from build123d import *

# Parameters (mm, degrees)
SKETCH2_OUTSIDE_W  = 34.928
SKETCH2_OUTSIDE_H  = 34.928
SKETCH2_OUTSIDE_R  = 3.81
CUT_EXTRUDE1_DEPTH = 0.5
CHAMFER1_SIZE2     = 2
CHAMFER1_SIZE      = 0.515


with BuildPart() as part:
    # Sketch1 → Revolve1 (revolve)
    with BuildSketch(Plane.XY, mode=Mode.PRIVATE) as revolve1_sk:
        with BuildLine():
            Line((0, 0), (64.25, 0))
            Line((64.25, 0), (64.25, 4.325))
            Line((64.25, 4.325), (56.25, 4.325))
            ThreePointArc((56.25, 4.325), (52.653126358, 4.994271197), (49.5377095, 6.9125))
            ThreePointArc((49.5377095, 6.9125), (46.422292643, 8.830728803), (42.825419001, 9.5))
            Line((42.825419001, 9.5), (9.5, 9.5))
            ThreePointArc((9.5, 9.5), (2.782485579, 6.717514421), (0, 0))
        make_face()
    revolve(revolve1_sk.sketch.rotate(Axis((71.903875566, 0, 0), (1, 0, 0)), 90), axis=Axis((71.903875566, 0, 0), (1, 0, 0)))

    # Sketch2 outside → Cut-Extrude1 (cut)
    with BuildSketch(Plane(origin=(64.25, 0, 0), x_dir=(0, 0, -1), z_dir=(1, 0, 0))):
        Rectangle(SKETCH2_OUTSIDE_W, SKETCH2_OUTSIDE_H)
        Circle(SKETCH2_OUTSIDE_R, mode=Mode.SUBTRACT)
    extrude(amount=-CUT_EXTRUDE1_DEPTH, mode=Mode.SUBTRACT)

    # Chamfer1
    chamfer1_edges = [part.edges().sort_by_distance(p)[0] for p in [
        (63.75, 0, -4.325),
    ]]
    chamfer1_side = [part.faces().sort_by_distance(p)[0] for p in [
        (63.75, 0, -4.3147),
    ]]
    chamfer(chamfer1_edges, length=CHAMFER1_SIZE - 0.0001, length2=CHAMFER1_SIZE2 - 0.0001, reference=chamfer1_side[0])  # a hair under: the kernel refuses the full size


solid = part.part
Part model, mm, in its own coordinate system. A direction names the side the tool comes from. Give positions to 0.01 mm unless a question says otherwise; leave off trailing zeros. Order: outer loops, then holes, each group sorted by start corner. A loop starts at its lowest first (then second) coordinate and runs counter-clockwise, first axis right, second up. Notation, with made-up numbers: (82, 22.5) - (137, 22.5) arc R4 ccw to (137, 26.5) - close; hole circle Ø5 at (17.5, -39). An arc over 180 degrees is marked (long way). One line per question, with ' | ' between items.
1. Drop flat-ended pins along their axis: P1, Ø1.5, axis at y = -0.5, z = 6.5, coming from the +X side; P2, Ø6, axis at y = -2.5, z = -5, coming from the -X side; P3, Ø1.5, axis at x = 31, z = 2, coming from the -Y side; P4, Ø8, axis at y = 3.5, z = -0.5, coming from the -X side. Give the stop position or say it passes through.
Filled in:
P1: x = 51.07 | P2: x = 0.36 | P3: y = -9.42 | P4: x = 0
2. Drill centre lines: probe 1 along Z at (x, y) = (38, 3.25); probe 2 along Z at (x, y) = (5.5, -0.25); probe 3 along X at (y, z) = (3.5, -1). Where is each one in solid material? Low to high.
Filled in:
probe 1: -8.93 to 8.93 | probe 2: -8.61 to 8.61 | probe 3: 0.73 to 64.25
3. Band-saw the part on A-A on x = 24. List the corners of the cut face in (y, z).
Filled in:
outline: circle Ø19 at (0, 0)
4. Which spindle directions (+Z, -Z, +X, -X, +Y, -Y) get a long thin tool onto all of the face, cutting with end or side? Do faces 1 (the face through (25.929, 9.274, -2.059)), 2 (the face through (64, -3.72, 0.83)). Say none if no direction does.
Filled in:
face 1: +X, -X | face 2: +X
5. Band-saw the part on B-B on x = 55.5. List the corners of the cut face in (y, z), then the cut area to 3 significant figures.
Filled in:
outline: circle Ø8.71 at (0, 0) | area: 59.5 mm²
